Geometry: final body of the model. Coordinates: model frame, mm. A direction names the side the tool comes from. Round coordinates to 2 decimals unless told otherwise and drop trailing zeros. Loops run counter-clockwise (first coordinate to the right, second up) from the corner with the lowest first, then second, coordinate; pieces in that order, holes last. Notation, with made-up numbers: (-16, -18.5) - (-3, -18.5) arc R34 cw to (-3, 20.5) - close; hole circle Ø3 at (54, 20). An arc over 180 degrees is marked (long way). Answer as a JSON object with one key per item and string values. Group by question number.
Item 1: First-contact query: pin 1 (7.5 mm diameter, centred on y = 2, z = 74.5, fed in from -X); pin 2 (10 mm diameter, centred on x = -9, z = 69, fed in from +Y); pin 3 (2 mm diameter, centred on x = 3.5, z = 73.5, fed in from -Y). Flat tips, straight axial feed; report the tip coordinate or a pass-through.
Item 2: Section C-C (y = 14). Return the cut outline in (x, z), plus the area to 3 significant figures.
Item 3: Reachability of faces 4 (the face through (23.1, 0, 77)), 5 (the face through (-27.65, -21, 77)), 6 (the face through (6.513, 25.343, 55.035)), 7 (the face through (27.65, -21, 77)), 8 (the face through (26.447, 26.509, 79.092)) from +Z, -Z, +X, -X, +Y, -Y: full face, straight path, thin tool, end or side. Return the list, or none.
Item 4: Draft query along X for faces 1 (the face through (0, -27.65, 24)), 2 (the face through (-27.65, 0, 77)), 3 (the face through (26.447, -26.509, 79.092)). Return one class per face: released by +X, released by -X, zero draft, split by the parting line, or undercut.
Item 5: Section A-A (y = 3). Return the cut outline in (x, z), plus the area to 3 significant figures.
Item 6: Line query: line 1 (X direction, y = 3, z = 82); line 2 (Z direction, x = 0, y = -26). Output: solid intervals per line, ascending.
Item 7: Section B-B (x = 0). Return the cut outline in (y, z).
```python
from build123d import *

# Parameters (mm, degrees)
F0_W     = 46.2
F0_H     = 46.2
F1_DEPTH = 156
F0_W_2   = 60
F0_H_2   = 60
F2_DEPTH = 4
F3_R     = 4
F4_R     = 2
F7_DEPTH = 80


with BuildPart() as f1:
    # F0 (on Top) → F1 (new body)
    with BuildSketch(Plane.XY):
        Polygon((27.65, 17.65), (27.65, 27.65), (-27.65, 27.65), (-27.65, 17.65), (-28.05, 17.65), (-28.05, 7.65), (-27.65, 7.65), (-27.65, -7.65), (-28.05, -7.65), (-28.05, -17.65), (-27.65, -17.65), (-27.65, -27.65), (-17.65, -27.65), (-17.65, -27.95), (-7.65, -27.95), (-7.65, -27.65), (7.65, -27.65), (7.65, -27.95), (17.65, -27.95), (17.65, -27.65), (27.65, -27.65), (27.65, -17.65), (28.05, -17.65), (28.05, -7.65), (27.65, -7.65), (27.65, 7.65), (28.05, 7.65), (28.05, 17.65), align=None)
        Rectangle(F0_W, F0_H, mode=Mode.SUBTRACT)
    extrude(amount=F1_DEPTH)

    # F0 (on Top) → F2 (join)
    with BuildSketch(Plane.XY):
        Rectangle(F0_W_2, F0_H_2)
        Polygon((-27.65, 27.65), (27.65, 27.65), (27.65, 17.65), (28.05, 17.65), (28.05, 7.65), (27.65, 7.65), (27.65, -7.65), (28.05, -7.65), (28.05, -17.65), (27.65, -17.65), (27.65, -27.65), (17.65, -27.65), (17.65, -27.95), (7.65, -27.95), (7.65, -27.65), (-7.65, -27.65), (-7.65, -27.95), (-17.65, -27.95), (-17.65, -27.65), (-27.65, -27.65), (-27.65, -17.65), (-28.05, -17.65), (-28.05, -7.65), (-27.65, -7.65), (-27.65, 7.65), (-28.05, 7.65), (-28.05, 17.65), (-27.65, 17.65), align=None, mode=Mode.SUBTRACT)
        Polygon((27.65, 17.65), (27.65, 27.65), (-27.65, 27.65), (-27.65, 17.65), (-28.05, 17.65), (-28.05, 7.65), (-27.65, 7.65), (-27.65, -7.65), (-28.05, -7.65), (-28.05, -17.65), (-27.65, -17.65), (-27.65, -27.65), (-17.65, -27.65), (-17.65, -27.95), (-7.65, -27.95), (-7.65, -27.65), (7.65, -27.65), (7.65, -27.95), (17.65, -27.95), (17.65, -27.65), (27.65, -27.65), (27.65, -17.65), (28.05, -17.65), (28.05, -7.65), (27.65, -7.65), (27.65, 7.65), (28.05, 7.65), (28.05, 17.65), align=None)
        Rectangle(F0_W, F0_H, mode=Mode.SUBTRACT)
    extrude(amount=-F2_DEPTH)

    # F3
    f3_edges = [f1.edges().sort_by_distance(p)[0] for p in [
        (-27.65, 27.65, 78),
        (-27.65, -27.65, 78),
        (27.65, -27.65, 78),
        (27.65, 27.65, 78),
        (30, 30, -2),
        (30, -30, -2),
        (-30, 30, -2),
        (-30, -30, -2),
    ]]
    fillet(f3_edges, radius=F3_R)

    # F4
    f4_edges = [f1.edges().sort_by_distance(p)[0] for p in [
        (30, 0, -4),
    ]]
    fillet(f4_edges, radius=F4_R)

    # F6 (on offset) → F7 (cut)
    with BuildSketch(Plane.XZ.offset(27.65)):
        with BuildLine():
            Line((-5.630705, 57.75), (-7.370688, 52.394882))
            ThreePointArc((-7.370688, 52.394882), (0, 42.25), (7.370688, 52.394882))
            Line((7.370688, 52.394882), (5.630705, 57.75))
            Line((5.630705, 57.75), (-5.630705, 57.75))
        make_face()
    extrude(amount=-F7_DEPTH, mode=Mode.SUBTRACT)


solid = f1.part
```
Values:
{
 "1": {"pin 1": "stops at x = -27.65", "pin 2": "stops at y = 27.65", "pin 3": "stops at y = -27.65"},
 "2": {"outline": "(-30, -2) arc R2 ccw to (-28, -4) - (-23.1, -4) - (-23.1, 156) - (-28.05, 156) - (-28.05, 0) - (-30, 0) - close; (23.1, -4) - (28, -4) arc R2 ccw to (30, -2) - (30, 0) - (28.05, 0) - (28.05, 156) - (23.1, 156) - close", "area": "1,600 mm^2"},
 "3": {"face 4": "+Z, -Z", "face 5": "+Z, -X, -Y", "face 6": "+Y, -Y", "face 7": "+Z, +X, -Y", "face 8": "+Z, +X, +Y"},
 "4": {"face 1": "undercut", "face 2": "released by -X", "face 3": "released by +X"},
 "5": {"outline": "(-30, -2) arc R2 ccw to (-28, -4) - (-23.1, -4) - (-23.1, 156) - (-27.65, 156) - (-27.65, 0) - (-30, 0) - close; (23.1, -4) - (28, -4) arc R2 ccw to (30, -2) - (30, 0) - (27.65, 0) - (27.65, 156) - (23.1, 156) - close", "area": "1,470 mm^2"},
 "6": {"line 1": "x = -27.65 to -23.1, 23.1 to 27.65", "line 2": "z = -4 to 42.25, 57.75 to 156"},
 "7": {"outline": "(-30, -2) arc R2 ccw to (-28, -4) - (-23.1, -4) - (-23.1, 42.25) - (-27.65, 42.25) - (-27.65, 0) - (-30, 0) - close; (-27.65, 57.75) - (-23.1, 57.75) - (-23.1, 156) - (-27.65, 156) - close; (23.1, -4) - (28, -4) arc R2 ccw to (30, -2) - (30, 0) - (27.65, 0) - (27.65, 42.25) - (23.1, 42.25) - close; (23.1, 57.75) - (27.65, 57.75) - (27.65, 156) - (23.1, 156) - close"}
}
